The figure shows three views and two pictorial views of one solid part (mm, origin at its lowest corner). Answer the questions. Round coordinates to 2 decimals unless told otherwise and drop trailing zeros. Write each loop counter-clockwise with the first axis right and the second up, starting at its lowest first coordinate (ties: lowest second). Pieces come first, ordered by that corner, then holes. Notation, with made-up numbers: M 51.5,88 L 57.5,88 A7 cw 57.5,96 Z; hole C 30,-26.5 d2. An arc over 180 degrees is marked long. Use one line per item in the form item = value. Start each with the question number.
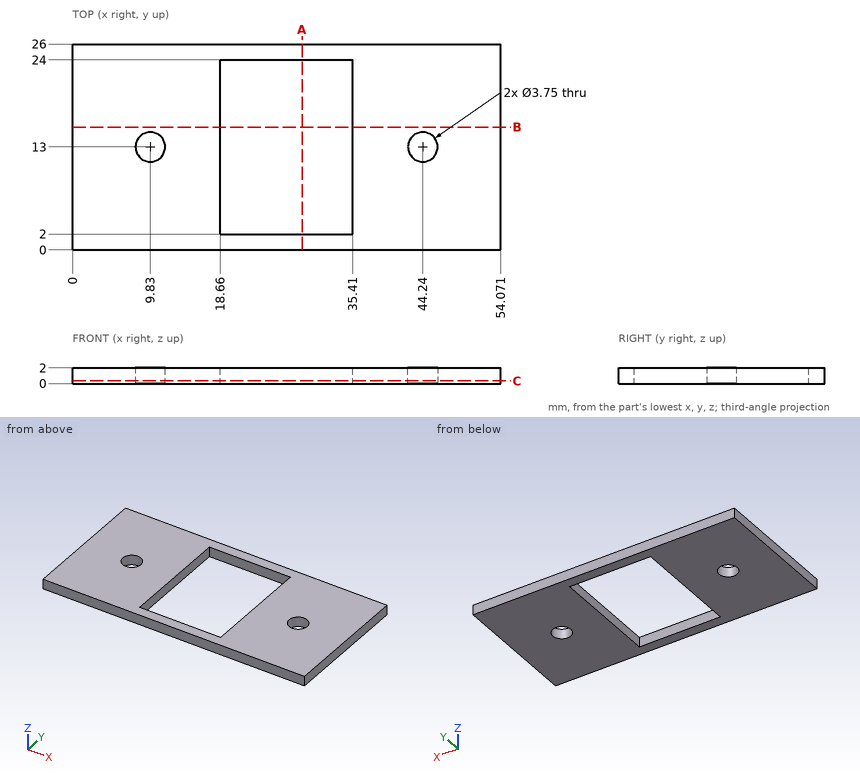
Q1. Find section C-C on z = 0.35. Count the separate pieces of the cut face and the enclosed holes in it.
Q2. Find section A-A on x = 29. Write down the section's boundary in (y, z).
Q3. Straight lines are drawn through the part: line 1 (X direction, y = 22.75, z = 1.4); line 2 (X direction, y = 13.75, z = 0.2); line 3 (Y direction, x = 30, z = 1.6). For each, find the intervals that lie inside material, in ascending order. Write a range as [from, to].
Q4. Find section B-B on y = 15.5. Write down the section's boundary in (x, z).
Response:
q1.separate_pieces = 1
q1.enclosed_holes = 3
q2.outline = M 0,0 L 2,0 L 2,2 L 0,2 Z; M 24,0 L 26,0 L 26,2 L 24,2 Z
q3.line_1 = [0, 18.66], [35.41, 54.07]
q3.line_2 = [0, 8.11], [11.55, 18.66], [35.41, 42.52], [45.96, 54.07]
q3.line_3 = [0, 2], [24, 26]
q4.outline = M 0,0 L 18.66,0 L 18.66,2 L 0,2 Z; M 35.41,0 L 54.07,0 L 54.07,2 L 35.41,2 Z
